from build123d import *

# Parameters (mm, degrees)
F0_W     = 172
F0_H     = 172
F1_DEPTH = 5
F2_W     = 15
F2_H     = 172
F3_DEPTH = 5


with BuildPart() as f1:
    # F0 (on Front) → F1 (new body)
    with BuildSketch(Plane.XZ):
        with Locations((0, -86)):
            Rectangle(F0_W, F0_H)
    extrude(amount=F1_DEPTH)

    # F2 (on face) → F3 (join)
    with BuildSketch(Plane(origin=(-86, 0, 0), x_dir=(0, -1, 0), z_dir=(-1, 0, 0))):
        with Locations((-2.5, -86)):
            Rectangle(F2_W, F2_H)
    extrude(amount=-F3_DEPTH)


solid = f1.part
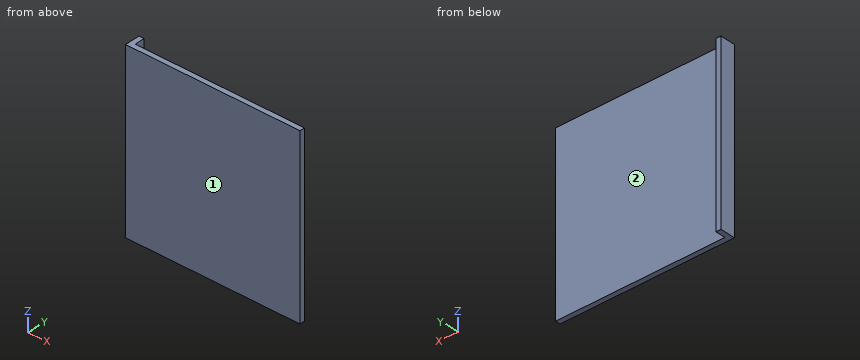
Work out the finished part from the listing and answer in its coordinate system (mm). Face numbers are marked on the shaded views. A direction names the side the tool comes from. Round coordinates to 2 decimals unless told otherwise and drop trailing zeros. Write each loop counter-clockwise with the first axis right and the second up, starting at its lowest first coordinate (ties: lowest second). Pieces come first, ordered by that corner, then holes. Notation, with made-up numbers: (-3.5, -25) -> (49.5, -25) arc R28 cw to (49.5, 1) -> close; hole circle Ø9 at (-27, 55). An arc over 180 degrees is marked (long way). Write each question's results on one line, items separated by ' | '.
Item 1: A flat-ended cylindrical pin translates along its axis: P1, Ø3, axis at y = 2.5, z = -76, coming from the +X side. Find the tip coordinate at first contact, or state that the pin passes through.
Result set:
P1: x = -81
Item 2: Which of the six approach directions +Z, -Z, +X, -X, +Y, -Y give full straight-line access (tool end or side, diameter ignored) to the marked faces 1 and 2?
Result set:
face 1: +Z, -Z, +X, -X, -Y | face 2: +Z, -Z, +X, +Y
Item 3: A cutting plane is placed at B-B, the plane y = 3. Determine the outline of the cut face in (x, z), plus the area to 3 significant figures.
Result set:
outline: (-86, -172) -> (-81, -172) -> (-81, 0) -> (-86, 0) -> close | area: 860 mm^2
Item 4: Find the intervals of material crossed by line 1 along Y through (x, z) = (49.5, -164); line 2 along X through (y, z) = (5.5, -10.5), in increasing order. Write a range as [from, to].
Result set:
line 1: [-5, 0] | line 2: [-86, -81]
Item 5: A cutting plane is placed at A-A, the plane x = -11.5. Determine the outline of the cut face in (y, z).
Result set:
outline: (-5, -172) -> (0, -172) -> (0, 0) -> (-5, 0) -> close
Item 6: A cutting plane is placed at C-C, the plane z = -10.5. Determine the outline of the cut face in (x, y).
Result set:
outline: (-86, -5) -> (86, -5) -> (86, 0) -> (-81, 0) -> (-81, 10) -> (-86, 10) -> close
